```python
from build123d import *

# Parameters (mm, degrees)
SKETCH1_W                              = 30
SKETCH1_H                              = 40
BODY_DEPTH                             = 5
CBORE_FOR_M2_HEX_HEAD_BOLT2_AT_2_COUNT = 2
CBORE_FOR_M2_HEX_HEAD_BOLT2_AT_2_PITCH = 15
LPATTERN1_COUNT                        = 2
LPATTERN1_PITCH                        = 13
FILLET1_R                              = 1


with BuildPart() as part:
    # Sketch1 → Body (new body, symmetric)
    with BuildSketch(Plane.XY):
        Rectangle(SKETCH1_W, SKETCH1_H)
    extrude(amount=BODY_DEPTH, both=True)

    # Sketch6 → CBORE for M2 Hex Head Bolt2 (revolve, cut)
    with BuildSketch(Plane(origin=(-7.5, 7.5, 5), x_dir=(0, -1, 0), z_dir=(1, 0, 0))):
        Polygon((0, 0), (0, 10.721032743), (1.2, 10), (1.2, 2), (2.2, 2), (2.2, 0), align=None)
    cbore_for_m2_hex_head_bolt2 = revolve(axis=Axis((-7.5, 7.5, 11.35), (0, 0, -1)), mode=Mode.SUBTRACT)

    # CBORE for M2 Hex Head Bolt2 at 2: CBORE for M2 Hex Head Bolt2 ×2
    with Locations(*[(i * CBORE_FOR_M2_HEX_HEAD_BOLT2_AT_2_PITCH, 0, 0) for i in range(1, CBORE_FOR_M2_HEX_HEAD_BOLT2_AT_2_COUNT)]):
        add(cbore_for_m2_hex_head_bolt2, mode=Mode.SUBTRACT)

    # LPattern1: CBORE for M2 Hex Head Bolt2 ×2
    with Locations(*[(0, -i * LPATTERN1_PITCH, 0) for i in range(1, LPATTERN1_COUNT)]):
        add(cbore_for_m2_hex_head_bolt2, mode=Mode.SUBTRACT)

    # LPattern1 copy 1 sketch → LPattern1 copy 1 (revolve, cut)
    with BuildSketch(Plane(origin=(7.5, -5.5, 5), x_dir=(0, -1, 0), z_dir=(1, 0, 0))):
        Polygon((0, 0), (0, 10.721032743), (1.2, 10), (1.2, 2), (2.2, 2), (2.2, 0), align=None)
    revolve(axis=Axis((7.5, -5.5, 11.35), (0, 0, -1)), mode=Mode.SUBTRACT)

    # Fillet1
    fillet1_edges = [part.edges().sort_by_distance(p)[0] for p in [
        (15, -20, 0),
        (-15, -20, 0),
        (-15, 20, 0),
        (15, 20, 0),
    ]]
    fillet(fillet1_edges, radius=FILLET1_R)


solid = part.part
```
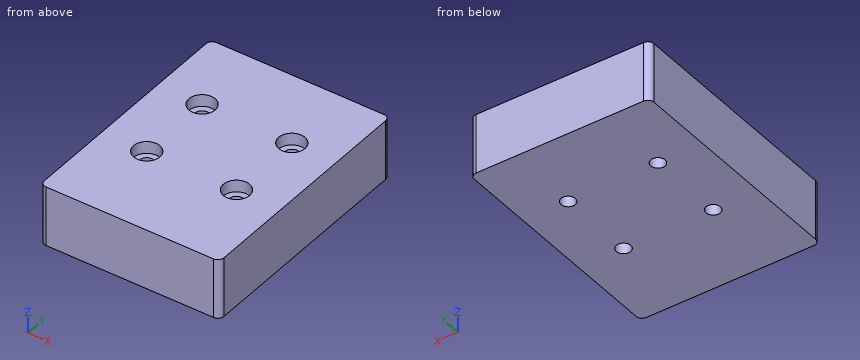
Work out the finished part from the listing and answer in its coordinate system (mm). Round coordinates to 2 decimals unless told otherwise and drop trailing zeros. Write each loop counter-clockwise with the first axis right and the second up, starting at its lowest first coordinate (ties: lowest second). Pieces come first, ordered by that corner, then holes.
1) A cutting plane is placed at C-C on z = 1.5. Determine the outline of the cut face in (x, y), and give its area (3 significant figures).
2) Consider probe 1 along Y at (x, z) = (-7.5, -2); probe 2 along Y at (x, z) = (-7.5, 3.4); probe 3 along X at (y, z) = (-5.5, 0.75). Determine where each line is inside the solid, lowest interval first.
3) Flat-ended cylindrical pins translate along their axes: P1, Ø3.5, axis at x = 8, y = -5, coming from the +Z side; P2, Ø3.5, axis at x = -7.5, y = -5.5, coming from the +Z side. Find the tip coordinate at first contact, or state that the pin passes through.
4) A cutting plane is placed at A-A on x = 7.5. Determine the outline of the cut face in (y, z), and give its area (3 significant figures).
5) A cutting plane is placed at B-B on y = -5.5. Determine the outline of the cut face in (x, z), and give its area (3 significant figures).
6) A cutting plane is placed at D-D on z = 3.5. Determine the outline of the cut face in (x, y).
Entries:
1. outline: (-15, -19) arc R1 ccw to (-14, -20) - (14, -20) arc R1 ccw to (15, -19) - (15, 19) arc R1 ccw to (14, 20) - (-14, 20) arc R1 ccw to (-15, 19) - close; hole circle Ø2.4 at (-7.5, -5.5); hole circle Ø2.4 at (-7.5, 7.5); hole circle Ø2.4 at (7.5, -5.5); hole circle Ø2.4 at (7.5, 7.5)
1. area: 1,180 mm2
2. probe 1: y = -20 to -6.7, -4.3 to 6.3, 8.7 to 20
2. probe 2: y = -20 to -7.7, -3.3 to 5.3, 9.7 to 20
2. probe 3: x = -15 to -8.7, -6.3 to 6.3, 8.7 to 15
3. P1: stops at z = 5
3. P2: stops at z = 3
4. outline: (-20, -5) - (-6.7, -5) - (-6.7, 3) - (-7.7, 3) - (-7.7, 5) - (-20, 5) - close; (-4.3, -5) - (6.3, -5) - (6.3, 3) - (5.3, 3) - (5.3, 5) - (-3.3, 5) - (-3.3, 3) - (-4.3, 3) - close; (8.7, -5) - (20, -5) - (20, 5) - (9.7, 5) - (9.7, 3) - (8.7, 3) - close
4. area: 344 mm2
5. outline: (-15, -5) - (-8.7, -5) - (-8.7, 3) - (-9.7, 3) - (-9.7, 5) - (-15, 5) - close; (-6.3, -5) - (6.3, -5) - (6.3, 3) - (5.3, 3) - (5.3, 5) - (-5.3, 5) - (-5.3, 3) - (-6.3, 3) - close; (8.7, -5) - (15, -5) - (15, 5) - (9.7, 5) - (9.7, 3) - (8.7, 3) - close
5. area: 244 mm2
6. outline: (-15, -19) arc R1 ccw to (-14, -20) - (14, -20) arc R1 ccw to (15, -19) - (15, 19) arc R1 ccw to (14, 20) - (-14, 20) arc R1 ccw to (-15, 19) - close; hole circle Ø4.4 at (-7.5, -5.5); hole circle Ø4.4 at (-7.5, 7.5); hole circle Ø4.4 at (7.5, -5.5); hole circle Ø4.4 at (7.5, 7.5)
